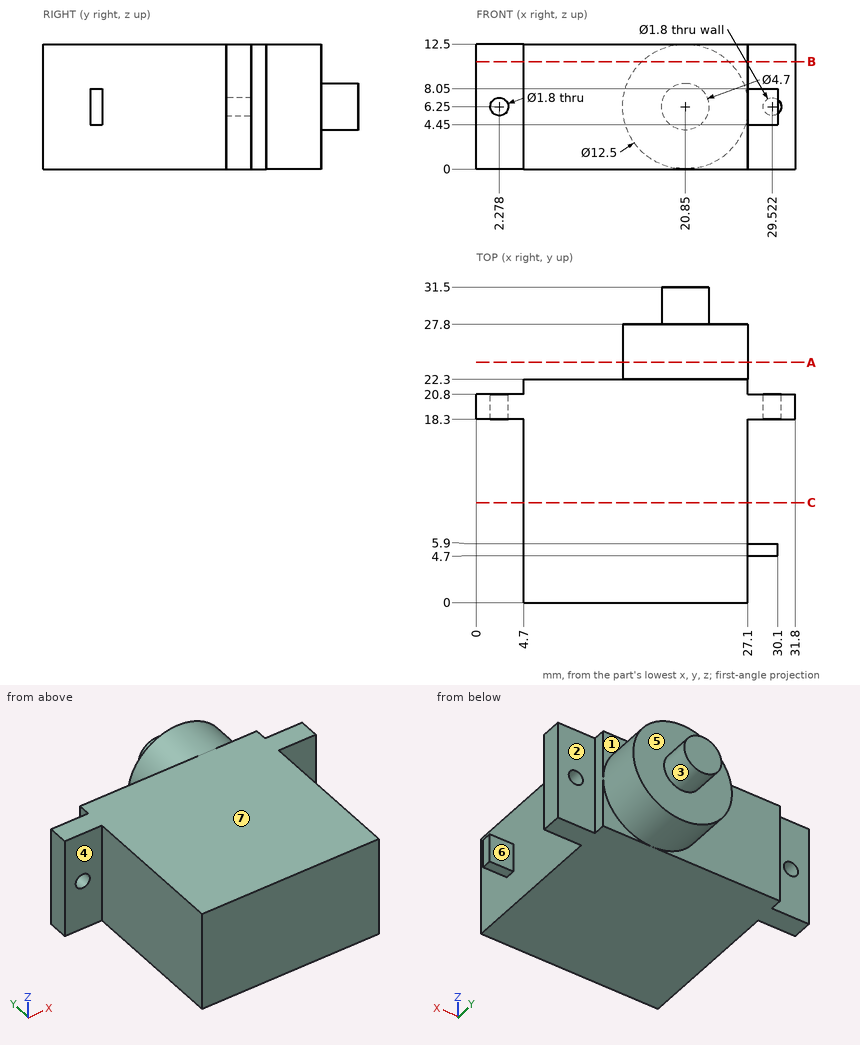
Geometry: see drawing. Coordinates: mm, zero at the bounding-box minimum. A direction names the side the tool comes from. Round coordinates to 2 decimals unless told otherwise and drop trailing zeros. Loops run counter-clockwise (first coordinate to the right, second up) from the corner with the lowest first, then second, coordinate; pieces in that order, holes last.
(1) Section query C-C (y = 10). Output: boundary loops of the cut face in (x, z), and give its area (3 significant figures).
From the geometry:
outline: (4.7, 0) - (27.1, 0) - (27.1, 12.5) - (4.7, 12.5) - close
area: 280 mm2
(2) Material intervals for probe 1 along X at (y, z) = (19.05, 6.25); probe 2 along X at (y, z) = (20.5, 6.5); probe 3 along X at (y, z) = (11, 6.5), sorted ascending.
From the geometry:
probe 1: x = 0 to 1.38, 3.18 to 28.62, 30.42 to 31.8
probe 2: x = 0 to 1.41, 3.14 to 28.66, 30.39 to 31.8
probe 3: x = 4.7 to 27.1
(3) Access query for the marked faces 1, 2, 3 and 4. Directions: +Z, -Z, +X, -X, +Y, -Y. A direction counts if a zero-diameter tool reaches every point of the face in a straight line with its end or side. Return the directions, or none.
From the geometry:
face 1: +Z, +X, +Y
face 2: +Z, -Z, +X, +Y
face 3: +Y
face 4: +Z, -Z, -X, -Y
(4) Section query A-A (y = 24). Output: boundary loops of the cut face in (x, z).
From the geometry:
outline: circle Ø12.5 at (20.85, 6.25)
(5) Pull-direction query (Y, two-part tool) for the marked faces 5, 6 and 7; classes: +Y half, -Y half, draft (parallel to the pull), parting line (faces both ways), or undercut.
From the geometry:
face 5: +Y half
face 6: undercut
face 7: draft
(6) Section query B-B (z = 10.75). Output: boundary loops of the cut face in (x, y), and give its area (3 significant figures).
From the geometry:
outline: (0, 18.3) - (4.7, 18.3) - (4.7, 0) - (27.1, 0) - (27.1, 18.3) - (31.8, 18.3) - (31.8, 20.8) - (27.1, 20.8) - (27.1, 22.3) - (25.19, 22.3) - (25.19, 27.8) - (16.51, 27.8) - (16.51, 22.3) - (4.7, 22.3) - (4.7, 20.8) - (0, 20.8) - close
area: 571 mm2
(7) Contact query for flat-ended pins moving along their axis: pin 1 Ø5 at (y, z) = (25.5, 8.5) entering from -X; pin 2 Ø3 at (y, z) = (20, 11) entering from -X; pin 3 Ø0.8 at (y, z) = (22, 6) entering from +X; pin 4 Ø1.4 at (x, z) = (2.28, 6.25) entering from -Y. Output: stop coordinate, or through.
From the geometry:
pin 1: stops at x = 14.6
pin 2: stops at x = 0
pin 3: stops at x = 27.1
pin 4: passes through
